from build123d import *

# Parameters (mm, degrees)
CHAMFER1_SIZE           = 0.5
CUT_EXTRUDE1_DEPTH      = 67.260395411
CUT_EXTRUDE1_DEPTH_BACK = 67.260395411
SKETCH3_R               = 0.45


with BuildPart() as part:
    # Sketch2 → Revolve1 (revolve)
    with BuildSketch(Plane(origin=(0, 0, 0), x_dir=(0, 0, -1), z_dir=(1, 0, 0)), mode=Mode.PRIVATE) as revolve1_sk:
        with BuildLine():
            Line((-29.233928571, 0), (65.5, 0))
            Line((65.5, 0), (66.2, 0))
            ThreePointArc((66.2, 0), (65.833883476, -0.883883476), (64.95, -1.25))
            Line((64.95, -1.25), (60.5, -1.25))
            Line((60.5, -1.25), (60.5, -1.5))
            Line((60.5, -1.5), (49.719225947, -1.5))
            Line((49.719225947, -1.5), (49.719225947, -2))
            Line((49.719225947, -2), (0, -2))
            Line((0, -2), (0, -1.25))
            Line((0, -1.25), (-5, -1.25))
            Line((-5, -1.25), (-30, -1.25))
            ThreePointArc((-30, -1.25), (-30.513084713, -0.716327439), (-30.7, 0))
            Line((-30.7, 0), (-29.233928571, 0))
        make_face()
    revolve(revolve1_sk.sketch.rotate(Axis((0, 0, 29.233928571), (0, 0, -1)), 270), axis=Axis((0, 0, 29.233928571), (0, 0, -1)))

    # Chamfer1
    chamfer1_edges = [part.edges().sort_by_distance(p)[0] for p in [
        (-2, 0, -49.719225947),
        (-2, 0, 0),
    ]]
    chamfer(chamfer1_edges, length=CHAMFER1_SIZE - 0.0001)  # a hair under: the kernel refuses the full size

    # Sketch3 → Cut-Extrude1 (cut, two sides: drawn at the far end of the back side and taken through both)
    with BuildSketch(Plane(origin=(0, 0, 0), x_dir=(0, 0, -1), z_dir=(1, 0, 0)).offset(-CUT_EXTRUDE1_DEPTH_BACK)):
        with Locations((-29.2, 0)):
            Circle(SKETCH3_R)
    extrude(amount=CUT_EXTRUDE1_DEPTH + CUT_EXTRUDE1_DEPTH_BACK, mode=Mode.SUBTRACT)


solid = part.part
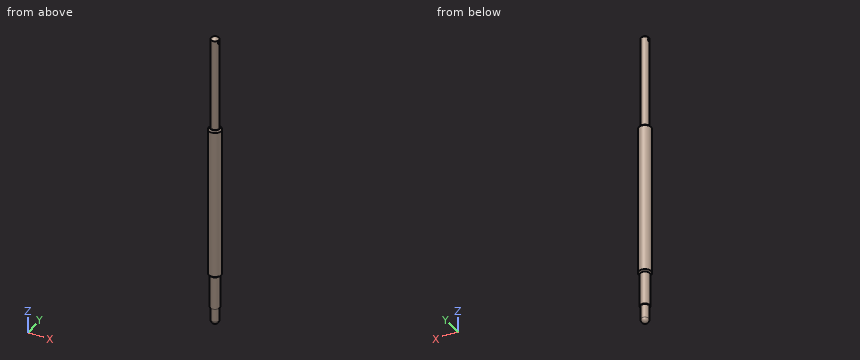
Verification items for the finished model (mm, model axes). Coordinates: 2 decimals unless noted, no trailing zeros. Order: outer loops, then holes, each group sorted by start corner. A loop starts at its lowest first (then second) coordinate and runs counter-clockwise, first axis right, second up.
Item 1: Section check B-B, the plane z = 8. Enter the section's corners in (x, y).
Filled in:
outline: circle Ø2.5 at (0, 0)
Item 2: Section check C-C, the plane z = -26. Enter the section's corners in (x, y).
Filled in:
outline: circle Ø4 at (0, 0)
Item 3: Material ranges on L1, parallel to Z at x = -0.2, y = 0; L2, parallel to Z at x = 1.25, y = 0.6; L3, parallel to X at y = -0.25, z = -19.5, recorded low to high.
Filled in:
L1: z = -66.18 to 28.75, 29.65 to 30.69
L2: z = -60.5 to 0
L3: x = -1.98 to 1.98
Item 4: Depth check by flat-ended pin: pin 1 (2 mm diameter, centred on y = -1, z = -50, fed in from +X); pin 2 (1 mm diameter, centred on y = 0, z = 3, fed in from +X). Enter the tip coordinate at first touch or a pass-through.
Filled in:
pin 1: stops at x = 1.96
pin 2: stops at x = 1.25
